Input: part model. Units: mm. Frame: model coordinates. Face numbers are marked on the shaded views. A direction names the side the tool comes from. Round coordinates to 2 decimals unless told otherwise and drop trailing zeros. Loops run counter-clockwise (first coordinate to the right, second up) from the corner with the lowest first, then second, coordinate; pieces in that order, holes last. Notation, with made-up numbers: M 40,-31 L 46,-31 A31 ccw 46,-2 Z; hole C -8,24 d11. An arc over 180 degrees is marked long. Put each result on its own line as item: value. Start each with the question number.
1) Line query: probe 1 along X at (y, z) = (-22.5, -20); probe 2 along X at (y, z) = (3.75, 24.5); probe 3 along Y at (x, z) = (-6, 4). Output: solid intervals per line, ascending.
2) Section B-B on x = 0. State how many separate pieces and enclosed holes the cut face has, plus the area to 3 significant figures.
3) Draft query along X for the marked faces 1, 2 and 3. Return one class per face: +X half, -X half, draft (parallel to the pull), parting line (faces both ways), or undercut.
4) Pin query (flat end, axial travel): pin 1 (1.8 mm diameter, centred on x = -29, z = -24.5, fed in from -Y); pin 2 (2 mm diameter, centred on x = 0, y = -16, fed in from +Z); pin 3 (1.2 mm diameter, centred on x = 0.5, y = -16, fed in from -Z); pin 4 (1.5 mm diameter, centred on y = 2.5, z = -18.5, fed in from +X). Return the tip coordinate at first contact, or that it passes through.
5) Reachability of the marked faces 4, 5, 6 and 7 from +Z, -Z, +X, -X, +Y, -Y: full face, straight path, thin tool, end or side. Return the list, or none.
6) Section D-D on z = 3.5. Output: boundary loops of the cut face in (x, y), plus the area to 3 significant figures.
7) Section C-C on x = -29. Output: boundary loops of the cut face in (y, z).
8) Section A-A on y = -10.5. Output: boundary loops of the cut face in (x, z).
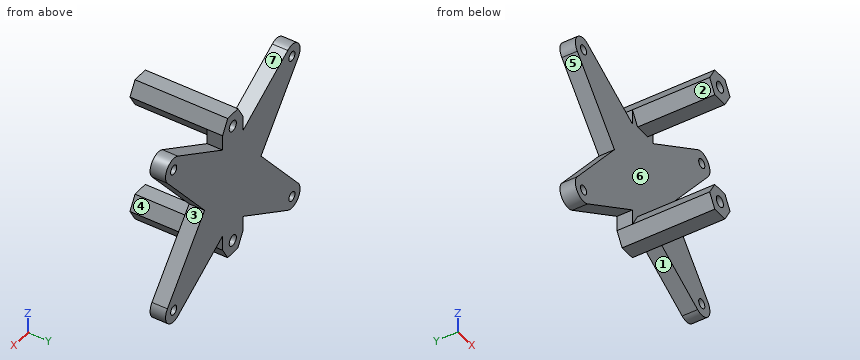
from build123d import *

# Parameters (mm, degrees)
BOSS_EXTRU_1_DEPTH      = 5
ESQUISSE2_R             = 1.5
ENL_V_MAT_EXTRU_2_DEPTH = 5
ESQUISSE4_R             = 1.75
BOSS_EXTRU_6_DEPTH      = 5
BOSS_EXTRU_7_START      = 14.5
ESQUISSE4_3_R           = 1.75
BOSS_EXTRU_7_DEPTH      = 14.5
BOSS_EXTRU_8_DEPTH      = 2.5
BOSS_EXTRU_10_START     = 25
ESQUISSE4_6_R           = 1.75
BOSS_EXTRU_10_DEPTH     = 8


with BuildPart() as part:
    # Esquisse1 → Boss.-Extru.1 (new body)
    with BuildSketch(Plane(origin=(0, 0, 0), x_dir=(1, 0, 0), z_dir=(0, 1, 0))):
        with BuildLine():
            Line((-13.840985932, 0), (-32.076386522, -21.943469936))
            ThreePointArc((-32.076386522, -21.943469936), (-32.047229987, -27.091213887), (-26.971076335, -27.947240746))
            Line((-26.971076335, -27.947240746), (0, -12.073021601))
            Line((0, -12.073021601), (26.971076335, -27.947240746))
            ThreePointArc((26.971076335, -27.947240746), (32.047229987, -27.091213887), (32.076386522, -21.943469936))
            Line((32.076386522, -21.943469936), (13.840985932, 0))
            Line((13.840985932, 0), (32.076386522, 21.943469936))
            ThreePointArc((32.076386522, 21.943469936), (32.047229987, 27.091213887), (26.971076335, 27.947240746))
            Line((26.971076335, 27.947240746), (0, 12.073021601))
            Line((0, 12.073021601), (-26.971076335, 27.947240746))
            ThreePointArc((-26.971076335, 27.947240746), (-32.047229987, 27.091213887), (-32.076386522, 21.943469936))
            Line((-32.076386522, 21.943469936), (-13.840985932, 0))
        make_face()
    extrude(amount=BOSS_EXTRU_1_DEPTH)

    # Esquisse2 → Enl_v. mat.-Extru.2 (cut)
    with BuildSketch(Plane(origin=(0, 5, 0), x_dir=(1, 0, 0), z_dir=(0, 1, 0))):
        with Locations(Location((-29, 24.5, 0), (0, 0, 270))):
            Circle(ESQUISSE2_R)
        with Locations(Location((29, 24.5, 0), (0, 0, 270))):
            Circle(ESQUISSE2_R)
        with Locations(Location((29, -24.5, 0), (0, 0, 270))):
            Circle(ESQUISSE2_R)
        with Locations(Location((-29, -24.5, 0), (0, 0, 270))):
            Circle(ESQUISSE2_R)
    extrude(amount=-ENL_V_MAT_EXTRU_2_DEPTH, mode=Mode.SUBTRACT)

    # Esquisse4 → Boss.-Extru.6 (add)
    # profile 1 of 4: a face of its own
    with BuildSketch(Plane.XZ):
        Polygon((2.5, -15.669872981), (5, -20), (5, -15.015844303), (0, -12.073021601), (-5, -15.015844303), (-5, -20), (-2.5, -15.669872981), align=None)
    # profile 2 of 4: a face of its own
    with BuildSketch(Plane.XZ):
        Polygon((-2.5, -24.330127019), (2.5, -24.330127019), (5, -20), (2.5, -15.669872981), (-2.5, -15.669872981), (-5, -20), align=None)
        with Locations(Location((0, -20, 0), (0, 0, 270))):
            Circle(ESQUISSE4_R, mode=Mode.SUBTRACT)
    # profile 3 of 4: a face of its own
    with BuildSketch(Plane.XZ):
        Polygon((-2.5, 15.669872981), (-5, 20), (-5, 15.015844303), (0, 12.073021601), (5, 15.015844303), (5, 20), (2.5, 15.669872981), align=None)
    # profile 4 of 4: a face of its own
    with BuildSketch(Plane.XZ):
        Polygon((-2.5, 15.669872981), (2.5, 15.669872981), (5, 20), (2.5, 24.330127019), (-2.5, 24.330127019), (-5, 20), align=None)
        with Locations(Location((0, 20, 0), (0, 0, 270))):
            Circle(ESQUISSE4_R, mode=Mode.SUBTRACT)
    extrude(amount=-BOSS_EXTRU_6_DEPTH)

    # Esquisse4_3 → Boss.-Extru.7 (add)
    # profile 1 of 2: a face of its own
    with BuildSketch(Plane.XZ.offset(BOSS_EXTRU_7_START)):
        Polygon((-2.5, 15.669872981), (2.5, 15.669872981), (5, 20), (2.5, 24.330127019), (-2.5, 24.330127019), (-5, 20), align=None)
        with Locations(Location((0, 20, 0), (0, 0, 270))):
            Circle(ESQUISSE4_3_R, mode=Mode.SUBTRACT)
    # profile 2 of 2: a face of its own
    with BuildSketch(Plane.XZ.offset(BOSS_EXTRU_7_START)):
        Polygon((-2.5, -24.330127019), (2.5, -24.330127019), (5, -20), (2.5, -15.669872981), (-2.5, -15.669872981), (-5, -20), align=None)
        with Locations(Location((0, -20, 0), (0, 0, 270))):
            Circle(ESQUISSE4_3_R, mode=Mode.SUBTRACT)
    extrude(amount=-BOSS_EXTRU_7_DEPTH)

    # Esquisse5 → Boss.-Extru.8 (add)
    # profile 1 of 2: a face of its own
    with BuildSketch(Plane.XZ.offset(14.5)):
        Polygon((5, 20), (2.5, 24.330127019), (-2.5, 24.330127019), (-5, 20), (-2.5, 15.669872981), (2.5, 15.669872981), align=None)
        Polygon((2.886751346, 20), (1.443375673, 22.5), (-1.443375673, 22.5), (-2.886751346, 20), (-1.443375673, 17.5), (1.443375673, 17.5), align=None, mode=Mode.SUBTRACT)
    # profile 2 of 2: a face of its own
    with BuildSketch(Plane.XZ.offset(14.5)):
        Polygon((5, -20), (2.5, -15.669872981), (-2.5, -15.669872981), (-5, -20), (-2.5, -24.330127019), (2.5, -24.330127019), align=None)
        Polygon((3.175426481, -20), (1.58771324, -17.25), (-1.58771324, -17.25), (-3.175426481, -20), (-1.58771324, -22.75), (1.58771324, -22.75), align=None, mode=Mode.SUBTRACT)
    extrude(amount=BOSS_EXTRU_8_DEPTH)

    # Esquisse4_6 → Boss.-Extru.10 (add)
    # profile 1 of 2: a face of its own
    with BuildSketch(Plane.XZ.offset(BOSS_EXTRU_10_START)):
        Polygon((-2.5, 15.669872981), (2.5, 15.669872981), (5, 20), (2.5, 24.330127019), (-2.5, 24.330127019), (-5, 20), align=None)
        with Locations(Location((0, 20, 0), (0, 0, 270))):
            Circle(ESQUISSE4_6_R, mode=Mode.SUBTRACT)
    # profile 2 of 2: a face of its own
    with BuildSketch(Plane.XZ.offset(BOSS_EXTRU_10_START)):
        Polygon((-2.5, -24.330127019), (2.5, -24.330127019), (5, -20), (2.5, -15.669872981), (-2.5, -15.669872981), (-5, -20), align=None)
        with Locations(Location((0, -20, 0), (0, 0, 270))):
            Circle(ESQUISSE4_6_R, mode=Mode.SUBTRACT)
    extrude(amount=-BOSS_EXTRU_10_DEPTH)


solid = part.part
Geometry results:
1. probe 1: x = -5 to -1.75, 1.75 to 5
1. probe 2: x = -33 to -30.5, -27.5 to -21.11, 21.11 to 27.5, 30.5 to 33
1. probe 3: y = 0 to 5
2. separate pieces: 3
2. enclosed holes: 0
2. area: 458 mm²
3. face 1: undercut
3. face 2: -X half
3. face 3: +X half
4. pin 1: passes through
4. pin 2: stops at z = 24.33
4. pin 3: stops at z = -24.33
4. pin 4: stops at x = 29.84
5. face 4: +X, -Y
5. face 5: -X, +Y, -Y
5. face 6: -Y
5. face 7: +Z, +Y, -Y
6. outline: M -16.75,0 L 16.75,0 L 16.75,5 L -16.75,5 Z
6. area: 167 mm²
7. outline: M 0,-28.5 L 5,-28.5 L 5,-26 L 0,-26 Z; M 0,-23 L 5,-23 L 5,-18.24 L 0,-18.24 Z; M 0,18.24 L 5,18.24 L 5,23 L 0,23 Z; M 0,26 L 5,26 L 5,28.5 L 0,28.5 Z
8. outline: M -5,-20 L -2.5,-24.33 L 2.5,-24.33 L 5,-20 L 2.5,-15.67 L -2.5,-15.67 Z; M -5,20 L -2.5,15.67 L 2.5,15.67 L 5,20 L 2.5,24.33 L -2.5,24.33 Z; hole C 0,-20 d3.5; hole C 0,20 d3.5
